Design review of the part built by this model. Coordinates are the model's own, in mm. A direction names the side the tool comes from. Coordinates: 2 decimals unless noted, no trailing zeros. Order: outer loops, then holes, each group sorted by start corner. A loop starts at its lowest first (then second) coordinate and runs counter-clockwise, first axis right, second up. Notation, with made-up numbers: (-28.75, 15) -> (-3.75, 15) arc R26 cw to (-3.75, 52) -> close; hole circle Ø8 at (-22.5, -13.75). An arc over 180 degrees is marked (long way). Write item = value, one per line.
```python
from build123d import *

# Parameters (mm, degrees)
F0_R     = 34.925
F0_R_2   = 5.35813
F1_DEPTH = 40.132
F2_DEPTH = 9.525
F4_R     = 12.4587
F5_DEPTH = 50.8
F6_R     = 5.35813
F7_DEPTH = 25.4
F8_R     = 5.35813
F9_DEPTH = 11.303


with BuildPart() as f1:
    # F0 (on Top) → F1 (new body)
    with BuildSketch(Plane.XY):
        Circle(F0_R)
        Circle(F0_R_2, mode=Mode.SUBTRACT)
    extrude(amount=F1_DEPTH)

    # F0 (on Top) → F2 (join)
    with BuildSketch(Plane.XY):
        Circle(F0_R_2)
    extrude(amount=F2_DEPTH)

    # F4 (on face) → F5 (join)
    with BuildSketch(Plane.XY):
        Circle(F4_R)
    extrude(amount=-F5_DEPTH)

    # F6 (on face) → F7 (cut)
    with BuildSketch(Plane(origin=(0, 0, -50.8), x_dir=(1, 0, 0), z_dir=(0, 0, -1))):
        Circle(F6_R)
    extrude(amount=-F7_DEPTH, mode=Mode.SUBTRACT)

    # F8 (on Top) → F9 (join)
    with BuildSketch(Plane.XY):
        Circle(F8_R)
    extrude(amount=F9_DEPTH)


solid = f1.part
```
(1) Insertion check: pin 1 (2 mm diameter, centred on x = 1, z = 29, fed in from +Y) (3 decimals); pin 2 (5 mm diameter, centred on x = -1.5, y = 15, fed in from -Z); pin 3 (6 mm diameter, centred on y = -12, z = 29.5, fed in from +X). Each pin has a flat end and moves straight along its axis. Give the tip position at first contact, or say it passes through.
Report:
pin_1 = 34.925
pin_2 = 0
pin_3 = 33.75
(2) We need section B-B (z = -39). Write out the cut boundary in (x, y).
Report:
outline = circle Ø24.92 at (0, 0); hole circle Ø10.72 at (0, 0)
(3) The part is to be moulded in two halves that separate along Y. For faces 1 (the cylindrical face through (2.472, -4.754, 25.516)), 2 (the cylindrical face through (-2.701, -12.162, -25.044)), 3 (the flat face through (0, -15, 0)), say which applies: released by +Y, released by -Y, zero draft, split by the parting line, or undercut.
Report:
face_1 = undercut
face_2 = split by the parting line
face_3 = zero draft
(4) We need section A-A (x = 0). Write out the cut boundary in (y, z) (3 decimals).
Report:
outline = (-34.925, 0) -> (-12.459, 0) -> (-12.459, -50.8) -> (-5.358, -50.8) -> (-5.358, -25.4) -> (5.358, -25.4) -> (5.358, -50.8) -> (12.459, -50.8) -> (12.459, 0) -> (34.925, 0) -> (34.925, 40.132) -> (5.358, 40.132) -> (5.358, 11.303) -> (-5.358, 11.303) -> (-5.358, 40.132) -> (-34.925, 40.132) -> close
(5) For L1, parallel to Y at x = 0, z = 32 (3 decimals); L2, parallel to Y at x = 0, z = -31; L3, parallel to Z at x = -15, y = 26, list the stretches that pass through material, from the lowest coordinate up.
Report:
L1 = -34.925 to -5.358, 5.358 to 34.925
L2 = -12.46 to -5.36, 5.36 to 12.46
L3 = 0 to 40.13
(6) We need section D-D (z = -2.5). Write out the cut boundary in (x, y), and give its area (3 significant figures).
Report:
outline = circle Ø24.92 at (0, 0)
area = 488 mm²
(7) For faces 4 (the cylindrical face through (-27.715, -21.251, 19.785)), 5 (the flat face through (0, 0, 11.303)), 6 (the cylindrical face through (2.472, 4.754, -38.278)), list the 3-axis set-ups (+Z, -Z, +X, -X, +Y, -Y) from which the entire face can be reached by the end or side of a thin tool; tool diameter is ignored.
Report:
face_4 = +Z, -Z
face_5 = +Z
face_6 = -Z
